```python
from build123d import *

# Parameters (mm, degrees)
PAD020_DEPTH    = 3
PAD021_DEPTH    = 2
CHAMFER028_SIZE = 1
POCKET031_DEPTH = 3
FILLET021_R     = 2
CHAMFER030_SIZE = 0.5
FILLET022_R     = 0.5


with BuildPart() as part:
    # Sketch055 → Pad020 (new body)
    with BuildSketch(Plane.XZ):
        with BuildLine():
            ThreePointArc((15.757359, 4.242641), (15.757359, -4.242641), (24.242641, -4.242641))
            Line((40, 11.514719), (24.242641, -4.242641))
            Line((40, 28.485281), (40, 11.514719))
            Line((15.757359, 4.242641), (40, 28.485281))
        make_face()
    extrude(amount=-PAD020_DEPTH)

    # Sketch056 (on Face6 of Pad020) → Pad021 (join)
    with BuildSketch(Plane(origin=(0, 3, 0), x_dir=(-1, 0, 0), z_dir=(0, 1, 0))):
        with BuildLine():
            Line((-40, 5.857864), (-40, 34.142136))
            Line((-40, 34.142136), (-12.928932, 7.071068))
            ThreePointArc((-27.071068, -7.071068), (-12.928932, -7.071068), (-12.928932, 7.071068))
            Line((-40, 5.857864), (-27.071068, -7.071068))
        make_face()
    extrude(amount=PAD021_DEPTH)

    # Chamfer028
    chamfer028_edges = [part.edges().sort_by_distance(p)[0] for p in [
        (33.535534, 5, -0.606602),
    ]]
    chamfer(chamfer028_edges, length=CHAMFER028_SIZE)

    # Sketch057 (on Face10 of Chamfer028) → Pocket031 (cut)
    with BuildSketch(Plane.XZ):
        with BuildLine():
            Line((40, 26.22254), (16.88873, 3.11127))
            ThreePointArc((16.88873, 3.11127), (16.88873, -3.11127), (23.11127, -3.11127))
            Line((40, 13.77746), (23.11127, -3.11127))
            Line((40, 26.22254), (40, 13.77746))
        make_face()
    extrude(amount=-POCKET031_DEPTH, mode=Mode.SUBTRACT)

    # Fillet021
    fillet021_edges = [part.edges().sort_by_distance(p)[0] for p in [
        (28.444365, 3, 14.666905),
    ]]
    fillet(fillet021_edges, radius=FILLET021_R)

    # Chamfer030
    chamfer030_edges = [part.edges().sort_by_distance(p)[0] for p in [
        (27.87868, 0, 16.363961),
    ]]
    chamfer(chamfer030_edges, length=CHAMFER030_SIZE)

    # Fillet022
    fillet022_edges = [part.edges().sort_by_distance(p)[0] for p in [
        (40, 0.5, 26.22254),
    ]]
    fillet(fillet022_edges, radius=FILLET022_R)


solid = part.part
```
Model file for the job. Use its own axes, mm. A direction names the side the tool comes from. Round coordinates to 2 decimals unless told otherwise and drop trailing zeros. Write each loop counter-clockwise with the first axis right and the second up, starting at its lowest first coordinate (ties: lowest second). Pieces come first, ordered by that corner, then holes. Notation, with made-up numbers: M 47,87 L 59,87 A23 ccw 59,126 Z; hole C 61.5,12.5 d8. An arc over 180 degrees is marked long. Put each result on its own line as item: value.
Item 1: Probe L1, parallel to X at y = 0.8, z = 1; L2, parallel to X at y = 1.7, z = 4; L3, parallel to Y at x = 38, z = 15.5. List the from-to ranges inside material, lowest first. Write a range as from..to.
Responses:
L1: 14.08..15.72, 27.22..29.49
L2: 15.53..17.96, 30.04..32.49
L3: 3..5
Item 2: Cut at A-A (z = 27). List the corners of the cut face in (x, y).
Responses:
outline: M 32.86,3 L 38.51,3 L 38.51,0.5 L 39.22,0 L 40,0 L 40,5 L 34.27,5 L 32.86,4 Z
Item 3: Tool access for faces 5 (the conical face through (13.67, 4.84, -6.62)), 6 (the flat face through (27.709, 1.732, 16.194)), 7 (the cylindrical face through (31.71, 2.43, 6.34)): list every direction of +Z, -Z, +X, -X, +Y, -Y with a clear straight run to the whole face (end or side of a thin tool).
Responses:
face 5: +Y
face 6: +Z, -X, -Y
face 7: -Y
Item 4: Flat gauge pins, fed straight in: P1, Ø12, axis at x = 28, z = 29.5, coming from the -Y side; P2, Ø1.5, axis at x = 22.5, z = -1.5, coming from the -Y side; P3, Ø1.5, axis at y = 3, z = 15, coming from the -X side. Where does each tip first touch, or does it go through?
Responses:
P1: y = 3
P2: y = 2.62
P3: x = 20.11
Item 5: Mould opens along X. For faces 1 (the flat face through (28.53, 0.49, 14.75)), 2 (the cylindrical face through (13.086, 3.493, -7.225)), 3 (the flat face through (33.626, 3.493, -0.516)), 4 (the flat face through (29, 5, 8)) say: +X half, -X half, draft (parallel to the pull), parting line (faces both ways), or undercut.
Responses:
face 1: undercut
face 2: parting line
face 3: +X half
face 4: draft
